Verification items for the finished model (mm, model axes). Face numbers are marked on the shaded views. A direction names the side the tool comes from. Give positions to 0.01 mm unless a question says otherwise; leave off trailing zeros. Loops run counter-clockwise (first coordinate to the right, second up) from the corner with the lowest first, then second, coordinate; pieces in that order, holes last. Notation, with made-up numbers: M 64.25,-24 L 119.25,-24 A12 cw 119.25,-11 Z; hole C 53,51.5 d7. An arc over 180 degrees is marked long. Write each question's results on one line, items separated by ' | '. Start each with the question number.
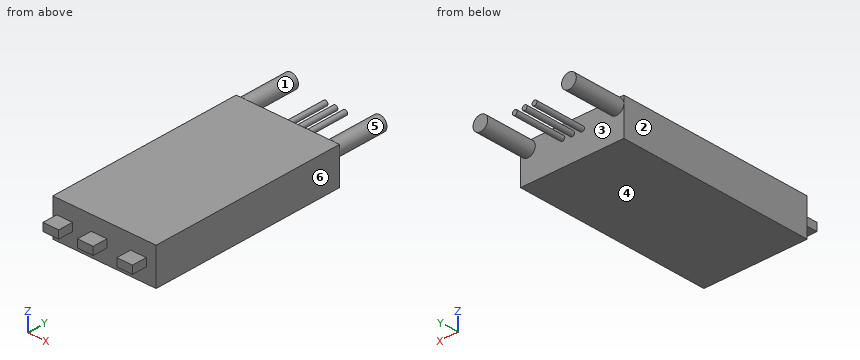
```python
from build123d import *

# Parameters (mm, degrees)
SKETCH1_W           = 40
SKETCH1_H           = 21
BOSS_EXTRUDE1_DEPTH = 3.75
SKETCH2_W           = 3
SKETCH2_H           = 3.2
BOSS_EXTRUDE2_DEPTH = 0.8
SKETCH3_R           = 1.5
SKETCH3_R_2         = 0.5
BOSS_EXTRUDE3_DEPTH = 10.366683148


with BuildPart() as part:
    # Sketch1 → Boss-Extrude1 (new, symmetric)
    with BuildSketch(Plane(origin=(0, 0, 0), x_dir=(0, 1, 0), z_dir=(0, 0, 1))):
        Rectangle(SKETCH1_W, SKETCH1_H)
    extrude(amount=BOSS_EXTRUDE1_DEPTH, both=True)

    # Sketch2 → Boss-Extrude2 (add, symmetric)
    with BuildSketch(Plane(origin=(0, 0, 0), x_dir=(0, 1, 0), z_dir=(0, 0, 1))):
        with Locations((-21.5, 8.1)):
            Rectangle(SKETCH2_W, SKETCH2_H)
        with Locations((-21.5, 1.1)):
            Rectangle(SKETCH2_W, SKETCH2_H)
        with Locations((-21.5, -6.9)):
            Rectangle(SKETCH2_W, SKETCH2_H)
    extrude(amount=BOSS_EXTRUDE2_DEPTH, both=True)

    # Sketch3 → Boss-Extrude3 (add)
    with BuildSketch(Plane(origin=(0, 20, 0), x_dir=(-1, 0, 0), z_dir=(0, 1, 0))):
        with Locations(Location((-9, 2.3, 0), (0, 0, 180))):
            Circle(SKETCH3_R)
        with Locations((9, 2.3)):
            Circle(SKETCH3_R)
        with Locations((0, 1.3)):
            Circle(SKETCH3_R_2)
        with Locations((2, 1.3)):
            Circle(SKETCH3_R_2)
        with Locations((-2, 1.3)):
            Circle(SKETCH3_R_2)
    extrude(amount=BOSS_EXTRUDE3_DEPTH)


solid = part.part
```
1. Release check for a two-part mould opening along X. For the marked faces 3, 4, 5 and 6 record: released by +X, released by -X, zero draft, split by the parting line, or undercut.
2. Depth check by flat-ended pin: pin 1 Ø6 at (x, y) = (2, 22) entering from +Z; pin 2 Ø0.8 at (y, z) = (-21.5, 0.5) entering from -X; pin 3 Ø1.5 at (x, z) = (7, 2.5) entering from -Y. Enter the tip coordinate at first touch or a pass-through.
3. Section check A-A, the plane x = -2. Record the boundary of the cut face in (y, z).
4. Section check D-D, the plane x = 2. Record the boundary of the cut face in (y, z), plus the area to 3 significant figures.
5. Section check B-B, the plane y = 21.5. Record the boundary of the cut face in (x, z), plus the area to 3 significant figures.
6. Thickness scan on probe 1 along Z at (x, y) = (5.5, -6.5); probe 2 along Y at (x, z) = (-0.5, -1.25); probe 3 along Y at (x, z) = (8.5, 3.5). Record the ranges inside material, lowest first.
7. Section check C-C, the plane z = 1.3. Record the boundary of the cut face in (x, y).
8. Set-up check for the marked faces 1 and 2: record each of +Z, -Z, +X, -X, +Y, -Y from which the full face is reachable in a straight line by a thin tool's end or side.
Filled sheet:
1) face 3: undercut | face 4: zero draft | face 5: undercut | face 6: released by +X
2) pin 1: z = 3.75 | pin 2: x = -9.7 | pin 3: y = -20
3) outline: M -23,-0.8 L -20,-0.8 L -20,-3.75 L 20,-3.75 L 20,0.8 L 30.37,0.8 L 30.37,1.8 L 20,1.8 L 20,3.75 L -20,3.75 L -20,0.8 L -23,0.8 Z
4) outline: M -20,-3.75 L 20,-3.75 L 20,0.8 L 30.37,0.8 L 30.37,1.8 L 20,1.8 L 20,3.75 L -20,3.75 Z | area: 310 mm2
5) outline: C -9,2.3 d3; C -2,1.3 d1; C 0,1.3 d1; C 2,1.3 d1; C 9,2.3 d3 | area: 16.5 mm2
6) probe 1: -3.75 to 3.75 | probe 2: -20 to 20 | probe 3: -20 to 30.37
7) outline: M -10.5,-20 L 10.5,-20 L 10.5,20 L 10.12,20 L 10.12,30.37 L 7.88,30.37 L 7.88,20 L 2.5,20 L 2.5,30.37 L 1.5,30.37 L 1.5,20 L 0.5,20 L 0.5,30.37 L -0.5,30.37 L -0.5,20 L -1.5,20 L -1.5,30.37 L -2.5,30.37 L -2.5,20 L -7.88,20 L -7.88,30.37 L -10.12,30.37 L -10.12,20 L -10.5,20 Z
8) face 1: +Y | face 2: +Z, -Z, -X, +Y, -Y
